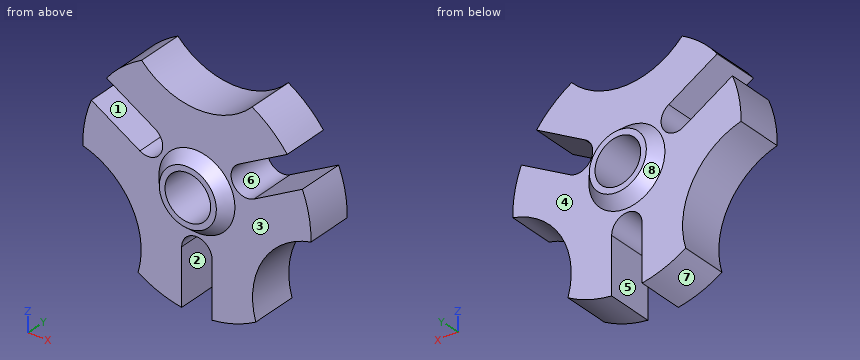
from build123d import *

# Parameters (mm, degrees)
SKETCH_1_R      = 6
EXTRUDE_2_DEPTH = 6


with BuildPart() as part:
    # 草图1 → 凸台-拉伸2 (new, symmetric)
    with BuildSketch(Plane(origin=(0, 0, 0), x_dir=(1, 0, 0), z_dir=(0, 1, 0))):
        with BuildLine():
            Line((-10.990381057, -10.964101615), (-23.748786379, -18.330170362))
            ThreePointArc((-23.748786379, -18.330170362), (-19.541660382, -22.76232654), (-14.523687548, -26.25))
            ThreePointArc((-14.523687548, -26.25), (0, -20), (14.523687548, -26.25))
            ThreePointArc((14.523687548, -26.25), (19.541660382, -22.76232654), (23.748786379, -18.330170362))
            Line((23.748786379, -18.330170362), (10.990381057, -10.964101615))
            ThreePointArc((10.990381057, -10.964101615), (9.526279442, -5.5), (14.990381057, -4.035898385))
            Line((14.990381057, -4.035898385), (27.748786379, -11.401967132))
            ThreePointArc((27.748786379, -11.401967132), (29.483583224, -5.542411054), (29.995010623, 0.547117627))
            ThreePointArc((29.995010623, 0.547117627), (17.320508076, 10), (15.471323075, 25.702882373))
            ThreePointArc((15.471323075, 25.702882373), (9.941922841, 28.304737593), (4, 29.732137495))
            Line((4, 29.732137495), (4, 15))
            ThreePointArc((4, 15), (0, 11), (-4, 15))
            Line((-4, 15), (-4, 29.732137495))
            ThreePointArc((-4, 29.732137495), (-9.941922841, 28.304737593), (-15.471323075, 25.702882373))
            ThreePointArc((-15.471323075, 25.702882373), (-17.320508076, 10), (-29.995010623, 0.547117627))
            ThreePointArc((-29.995010623, 0.547117627), (-29.483583224, -5.542411054), (-27.748786379, -11.401967132))
            Line((-27.748786379, -11.401967132), (-14.990381057, -4.035898385))
            ThreePointArc((-14.990381057, -4.035898385), (-9.526279442, -5.5), (-10.990381057, -10.964101615))
        make_face()
        with Locations(Location((0, 0, 0), (0, 0, 270))):
            Circle(SKETCH_1_R, mode=Mode.SUBTRACT)
    extrude(amount=EXTRUDE_2_DEPTH, both=True)

    # 草图3 → 旋转2 (revolve)
    with BuildSketch(Plane(origin=(0, 0, 0), x_dir=(0, 0, -1), z_dir=(1, 0, 0))):
        Polygon((-10, 6), (-7.5, 9), (-6, 9), (-6, 6), align=None)
    revolve_2 = revolve(axis=Axis((0, 16.131008677, 0), (0, -1, 0)))

    # 镜向2: 旋转2 across plane
    add(revolve_2.mirror(Plane.ZX))


solid = part.part
Work out the finished part from the listing and answer in its coordinate system (mm). Face numbers are marked on the shaded views. A direction names the side the tool comes from. Give positions to 0.01 mm unless a question says otherwise; leave off trailing zeros. Order: outer loops, then holes, each group sorted by start corner. A loop starts at its lowest first (then second) coordinate and runs counter-clockwise, first axis right, second up. Notation, with made-up numbers: (-21.75, 58) - (35.25, 58) arc R29 ccw to (35.25, 83) - close; hole circle Ø2 at (80, 62.25). An arc over 180 degrees is marked (long way). Answer as CSV lines item,"result". Start each with the question number.
Q1. Given pin 1 Ø10 at (y, z) = (-1.5, -10) entering from +X; pin 2 Ø3.5 at (y, z) = (-1.5, -23) entering from +X; pin 3 Ø2 at (x, z) = (1, 12) entering from +Y; pin 4 Ø10 at (x, y) = (19, 7) entering from +Z, each flat-ended and moving along its own axis, determine where each tip first touches the part or whether it passes through.
Q2. The part is cut by section C-C (z = -14). Write down the section's boundary in (x, y).
Q3. Find the intervals of material crossed by L1, parallel to Z at x = 0, y = -1.5; L2, parallel to X at y = 3.25, z = 11; L3, parallel to X at y = 1, z = 0, in increasing order. Write a range as [from, to].
Q4. The mould has two halves that part along X. Classify the marked faces 5, 6, 7 and 8: +X half, -X half, draft (parallel to the pull), parting line (faces both ways), or undercut.
Q5. The part is cut by section B-B (y = 3.75). Write down the section's boundary in (x, z), then the cut area to 3 significant figures.
Q6. The part is cut by section D-D (x = -22). Write down the section's boundary in (y, z), then the cut area to 3 significant figures.
Q7. The part is cut by section A-A (x = 0). Write down the section's boundary in (y, z), then the cut area to 3 significant figures.
Q8. For the marked faces 1, 2, 3 and 4, determine the directions among +Z, -Z, +X, -X, +Y, -Y from which every point of the face is accessible in a straight line to the end or side of a thin tool.
Check result:
1,pin 1,"stops at x = 21.41"
1,pin 2,"stops at x = 15.21"
1,pin 3,"stops at y = 6"
1,pin 4,"stops at z = 26.25"
2,outline,"(-15.56, -6) - (-3.87, -6) - (-3.87, 6) - (-15.56, 6) - close; (3.87, -6) - (15.56, -6) - (15.56, 6) - (3.87, 6) - close"
3,L1,"z = [-11, -6], [6, 20]"
3,L2,"x = [-27.91, -27.05], [-11.05, 11.05], [27.05, 27.91]"
3,L3,"x = [-30, -6], [6, 30]"
4,face 5,"undercut"
4,face 6,"undercut"
4,face 7,"-X half"
4,face 8,"parting line"
5,outline,"(-30, -0.55) arc R20 cw to (-15.47, -25.7) arc R30 ccw to (-4, -29.73) - (-4, -15) arc R4 cw to (4, -15) - (4, -29.73) arc R30 ccw to (15.47, -25.7) arc R20 cw to (30, -0.55) arc R30 ccw to (27.75, 11.4) - (14.99, 4.04) arc R4 cw to (10.99, 10.96) - (23.75, 18.33) arc R30 ccw to (14.52, 26.25) arc R20 cw to (-14.52, 26.25) arc R30 ccw to (-23.75, 18.33) - (-10.99, 10.96) arc R4 cw to (-14.99, 4.04) - (-27.75, 11.4) arc R30 ccw to start; hole circle Ø12 at (0, 0)"
5,area,"1,680 mm²"
6,outline,"(-6, -4.5) - (6, -4.5) - (6, 8.08) - (-6, 8.08) - close; (-6, 17.32) - (6, 17.32) - (6, 20.4) - (-6, 20.4) - close"
6,area,"188 mm²"
7,outline,"(-9, -7.5) - (-6, -10) - (-6, -11) - (6, -11) - (6, -10) - (9, -7.5) - (9, -6) - (-9, -6) - close; (-9, 6) - (9, 6) - (9, 7.5) - (6, 10) - (6, 20) - (-6, 20) - (-6, 10) - (-9, 7.5) - close"
7,area,"261 mm²"
8,face 1,"+Y, -Y"
8,face 2,"-Z, +Y, -Y"
8,face 3,"-Y"
8,face 4,"+Y"
